The listing builds one solid part. Answer for the finished solid, in the listing's coordinates (mm). Face numbers are marked on the shaded views. A direction names the side the tool comes from. Give positions to 0.01 mm unless a question says otherwise; leave off trailing zeros. Write each loop counter-clockwise with the first axis right and the second up, starting at its lowest first coordinate (ties: lowest second). Pieces come first, ordered by that corner, then holes. Notation, with made-up numbers: (48.5, -39) - (104.5, -39) arc R9 ccw to (104.5, -28) - close; hole circle Ø5 at (-2, -39.75). An arc over 180 degrees is marked (long way). One line per question, with ' | ' between items. Start each with the question number.
1. For the marked faces 4, 5 and 6, determine the directions among +Z, -Z, +X, -X, +Y, -Y from which every point of the face is accessible in a straight line to the end or side of a thin tool.
2. Find the intervals of material crossed by L1, parallel to Y at x = -11.3, z = 0.25; L2, parallel to Y at x = 10, z = 0; L3, parallel to X at y = -24, z = -0.1, in increasing order. Write a range as from..to.
3. A cutting plane is placed at D-D (y = 0.9). Determine the outline of the cut face in (x, z).
4. The mould has two halves that part along X. Classify the marked faces 1, 2 and 3: +X half, -X half, draft (parallel to the pull), parting line (faces both ways), or undercut.
5. A cutting plane is placed at C-C (z = -0.8). Determine the outline of the cut face in (x, y).
6. Given P1, Ø3.5, axis at x = 4.3, y = 0, coming from the -Z side; P2, Ø0.9, axis at x = -5.5, z = 0, coming from the -Y side; P3, Ø1.5, axis at y = -21, z = 0, coming from the +X side; P4, Ø1.5, axis at y = -23, z = -0.5, coming from the -X side, each flat-ended and moving along its own axis, determine where each tip first touches the part or whether it passes through.
7. A cutting plane is placed at B-B (y = -20). Determine the outline of the cut face in (x, z).
8. A cutting plane is placed at A-A (x = -11.3). Determine the outline of the cut face in (y, z), then the cut area to 3 significant figures.
```python
from build123d import *

# Parameters (mm, degrees)
BOSS_EXTRUDE1_DEPTH = 1.5
FILLET1_R           = 4
SKETCH2_R           = 4.1
SKETCH2_R_2         = 2.1
CUT_EXTRUDE1_DEPTH  = 39.103674364


with BuildPart() as part:
    # Sketch1 → Boss-Extrude1 (new, symmetric)
    with BuildSketch(Plane.XY):
        with BuildLine():
            Line((13.3, 10), (-13.3, 10))
            ThreePointArc((-13.3, 10), (-23.3, 0), (-13.3, -10))
            Line((-13.3, -10), (1.45, -10))
            Line((1.45, -10), (1.45, -30))
            Line((1.45, -30), (21.45, -30))
            Line((21.45, -30), (21.45, -5.794609564))
            ThreePointArc((21.45, -5.794609564), (22.186678109, 4.585515476), (13.3, 10))
        make_face()
    extrude(amount=BOSS_EXTRUDE1_DEPTH, both=True)

    # Fillet1
    fillet1_edges = [part.edges().sort_by_distance(p)[0] for p in [
        (21.45, -5.794609564, 0),
        (21.45, -30, 0),
        (1.45, -30, 0),
        (1.45, -10, 0),
    ]]
    fillet(fillet1_edges, radius=FILLET1_R)

    # Sketch2 → Cut-Extrude1 (cut, through all)
    with BuildSketch(Plane.XY.offset(1.5)):
        with Locations((-11.3, 0.9)):
            Circle(SKETCH2_R)
        with Locations((4.3, 0)):
            Circle(SKETCH2_R_2)
        with Locations((17.3, 0)):
            Circle(SKETCH2_R_2)
        with BuildLine():
            Line((8.45, -17.25), (14.45, -17.25))
            ThreePointArc((14.45, -17.25), (17.2, -20), (14.45, -22.75))
            Line((14.45, -22.75), (8.45, -22.75))
            ThreePointArc((8.45, -22.75), (5.7, -20), (8.45, -17.25))
        make_face()
    extrude(amount=-CUT_EXTRUDE1_DEPTH, mode=Mode.SUBTRACT)


solid = part.part
```
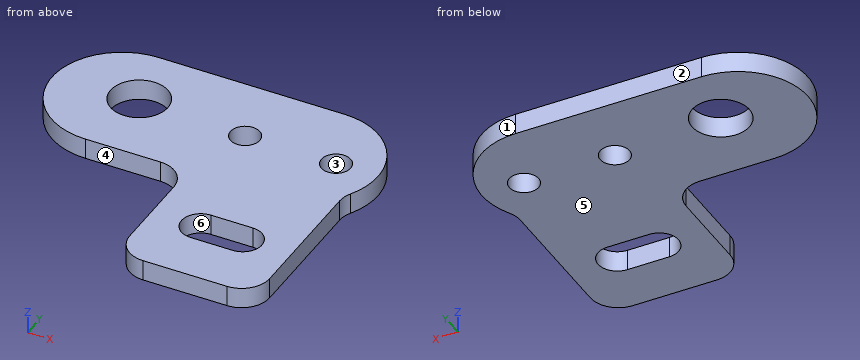
Determined:
1) face 4: +Z, -Z, -X, -Y | face 5: -Z, +X, -X, +Y, -Y | face 6: +Z, -Z
2) L1: -10..-3.2, 5..10 | L2: -30..-22.75, -17.25..10 | L3: 1.45..21.45
3) outline: (-23.26, -1.5) - (-15.4, -1.5) - (-15.4, 1.5) - (-23.26, 1.5) - close; (-7.2, -1.5) - (2.4, -1.5) - (2.4, 1.5) - (-7.2, 1.5) - close; (6.2, -1.5) - (15.4, -1.5) - (15.4, 1.5) - (6.2, 1.5) - close; (19.2, -1.5) - (23.26, -1.5) - (23.26, 1.5) - (19.2, 1.5) - close
4) face 1: +X half | face 2: draft | face 3: undercut
5) outline: (-13.3, -10) - (-2.55, -10) arc R4 cw to (1.45, -14) - (1.45, -26) arc R4 ccw to (5.45, -30) - (17.45, -30) arc R4 ccw to (21.45, -26) - (21.45, -6.96) arc R4 cw to (21.98, -4.97) arc R10 ccw to (13.3, 10) - (-13.3, 10) arc R10 ccw to start; hole circle Ø8.2 at (-11.3, 0.9); hole circle Ø4.2 at (4.3, 0); hole (8.45, -22.75) - (14.45, -22.75) arc R2.75 ccw to (14.45, -17.25) - (8.45, -17.25) arc R2.75 ccw to start; hole circle Ø4.2 at (17.3, 0)
6) P1: through | P2: y = -10 | P3: x = 21.45 | P4: x = 1.45
7) outline: (1.45, -1.5) - (5.7, -1.5) - (5.7, 1.5) - (1.45, 1.5) - close; (17.2, -1.5) - (21.45, -1.5) - (21.45, 1.5) - (17.2, 1.5) - close
8) outline: (-10, -1.5) - (-3.2, -1.5) - (-3.2, 1.5) - (-10, 1.5) - close; (5, -1.5) - (10, -1.5) - (10, 1.5) - (5, 1.5) - close | area: 35.4 mm2
